```python
from build123d import *

# Parameters (mm, degrees)
SKETCH1_R           = 1.55
BOSS_EXTRUDE1_DEPTH = 3
SKETCH2_R           = 1.55
BOSS_EXTRUDE2_DEPTH = 3
SKETCH3_R           = 1.55
BOSS_EXTRUDE3_DEPTH = 3


with BuildPart() as part:
    # Sketch1 → Boss-Extrude1 (new body)
    with BuildSketch(Plane.XY):
        with BuildLine():
            ThreePointArc((89.55, -5), (85, -0.45), (80.45, -5))
            Line((80.45, -5), (80.45, -11))
            Line((80.45, -11), (89.55, -11.011788251))
            Line((89.55, -11.011788251), (89.55, -5))
        make_face()
        with Locations((85, -5)):
            Circle(SKETCH1_R, mode=Mode.SUBTRACT)
    extrude(amount=BOSS_EXTRUDE1_DEPTH)



with BuildPart() as body_2:
    # Sketch2 → Boss-Extrude2 (new body)
    with BuildSketch(Plane(origin=(0, 0, -7), x_dir=(-1, 0, 0), z_dir=(0, 0, -1))):
        with BuildLine():
            Line((-89.55, -11.011788251), (-80.45, -11))
            Line((-80.45, -11), (-80.45, -5))
            ThreePointArc((-80.45, -5), (-85, -0.45), (-89.55, -5))
            Line((-89.55, -5), (-89.55, -11.011788251))
        make_face()
        with Locations((-85, -5)):
            Circle(SKETCH2_R, mode=Mode.SUBTRACT)
    extrude(amount=BOSS_EXTRUDE2_DEPTH)


with BuildPart() as part_1:
    add(part.part)

    add(body_2.part)  # Boss-Extrude3 merges body 2
    # Sketch3 → Boss-Extrude3 (add)
    with BuildSketch(Plane(origin=(-0.014114508, -10.895765801, 0), x_dir=(0.999999161, -0.001295411, 0), z_dir=(-0.001295411, -0.999999161, 0))):
        with BuildLine():
            Line((89.564189657, 3), (80.464182022, 3))
            Line((80.464182022, 3), (80.464182022, -10))
            Line((80.464182022, -10), (89.564189657, -10))
            Line((89.564189657, -10), (96.025380607, -7.808993039))
            ThreePointArc((96.025380607, -7.808993039), (99.114189657, -3.5), (96.025380607, 0.808993039))
            Line((96.025380607, 0.808993039), (89.564189657, 3))
        make_face()
        with Locations((94.564189657, -3.5)):
            Circle(SKETCH3_R, mode=Mode.SUBTRACT)
    extrude(amount=BOSS_EXTRUDE3_DEPTH)


solid = part_1.part
```
Here's how the part is built. I have some questions about the finished solid (model axes, mm). A direction names the side the tool comes from. Coordinates: 2 decimals unless noted, no trailing zeros. Order: outer loops, then holes, each group sorted by start corner. A loop starts at its lowest first (then second) coordinate and runs counter-clockwise, first axis right, second up. Notation, with made-up numbers: (7.5, 80) -> (26.5, 80) arc R21 cw to (26.5, 117) -> close; hole circle Ø8 at (28, 6.25). An arc over 180 degrees is marked (long way). Return JSON: item names as keys, results as strings.
1) I'm going to push flat-ended pins straight in: P1, Ø4, axis at x = 85, y = -5, coming from the +Z side; P2, Ø0.9, axis at y = -8.5, z = -9, coming from the -X side; P3, Ø1.5, axis at x = 91, y = -7.5, coming from the +Z side; P4, Ø1.5, axis at x = 83, z = -0.5, coming from the +Y side. Where does each tip first touch, or does it pass through?
Conclusion:
{"P1": "stops at z = 3", "P2": "stops at x = 80.45", "P3": "passes through", "P4": "stops at y = -0.68"}
2) If we section it at C-C on y = -6: List the corners of the cut face in (x, z) for me, plus the area to 3 significant figures.
Conclusion:
{"outline": "(80.45, -10) -> (83.82, -10) -> (83.82, -7) -> (80.45, -7) -> close; (80.45, 0) -> (83.82, 0) -> (83.82, 3) -> (80.45, 3) -> close; (86.18, -10) -> (89.55, -10) -> (89.55, -7) -> (86.18, -7) -> close; (86.18, 0) -> (89.55, 0) -> (89.55, 3) -> (86.18, 3) -> close", "area": "40.4 mm²"}
3) If we section it at A-A on y = -7.5: List the corners of the cut face in (x, z) for me, plus the area to 3 significant figures.
Conclusion:
{"outline": "(80.45, -10) -> (89.55, -10) -> (89.55, -7) -> (80.45, -7) -> close; (80.45, 0) -> (89.55, 0) -> (89.55, 3) -> (80.45, 3) -> close", "area": "54.6 mm²"}
4) On a 3-axis mill with a long thin cutter (end or side, diameter ignored), from which of +Z, -Z, +X, -X, +Y, -Y can I reach the whole of each face in a straight line? I mean faces 4 (the flat face through (85, -7, -7)), 5 (the cylindrical face through (83.522, -4.534, -8.479)), 6 (the flat face through (89.55, -8, -8)). Say none if no direction works.
Conclusion:
{"face 4": "+X, -X, +Y", "face 5": "+Z, -Z", "face 6": "+Z, -Z, +X, +Y"}
5) If we section it at D-D on z = 1.75: List the corners of the cut face in (x, y) for me.
Conclusion:
{"outline": "(80.45, -14) -> (93.23, -14.02) -> (93.24, -11.02) -> (89.55, -11.01) -> (89.55, -5) arc R4.55 ccw to (80.45, -5) -> (80.45, -11) -> close; hole circle Ø3.1 at (85, -5)"}
6) Thinking about a two-plate mould opening in Z: for faces 1 (the cylindrical face through (84.9, -0.45, -8.48)), 2 (the flat face through (85, -7, -10)), 3 (the flat face through (85, -7, 0)), which applies, +Z half, -Z half, draft (parallel to the pull), parting line (faces both ways), or undercut?
Conclusion:
{"face 1": "draft", "face 2": "-Z half", "face 3": "undercut"}
7) If we section it at B-B on x = 85: List the corners of the cut face in (y, z) for me, plus the area to 3 significant figures.
Conclusion:
{"outline": "(-14.01, -10) -> (-6.55, -10) -> (-6.55, -7) -> (-11.01, -7) -> (-11.01, 0) -> (-6.55, 0) -> (-6.55, 3) -> (-14.01, 3) -> close; (-3.45, -10) -> (-0.45, -10) -> (-0.45, -7) -> (-3.45, -7) -> close; (-3.45, 0) -> (-0.45, 0) -> (-0.45, 3) -> (-3.45, 3) -> close", "area": "83.7 mm²"}
8) If I drill on probe 1 along Y at (x, z) = (85, -7.9); probe 2 along Z at (x, y) = (87, -5.25); probe 3 along X at (y, z) = (-6.75, 0.75), over which ranges is the centre line in solid material (lowest first)?
Conclusion:
{"probe 1": "y = -14.01 to -6.55, -3.45 to -0.45", "probe 2": "z = -10 to -7, 0 to 3", "probe 3": "x = 80.45 to 89.55"}
